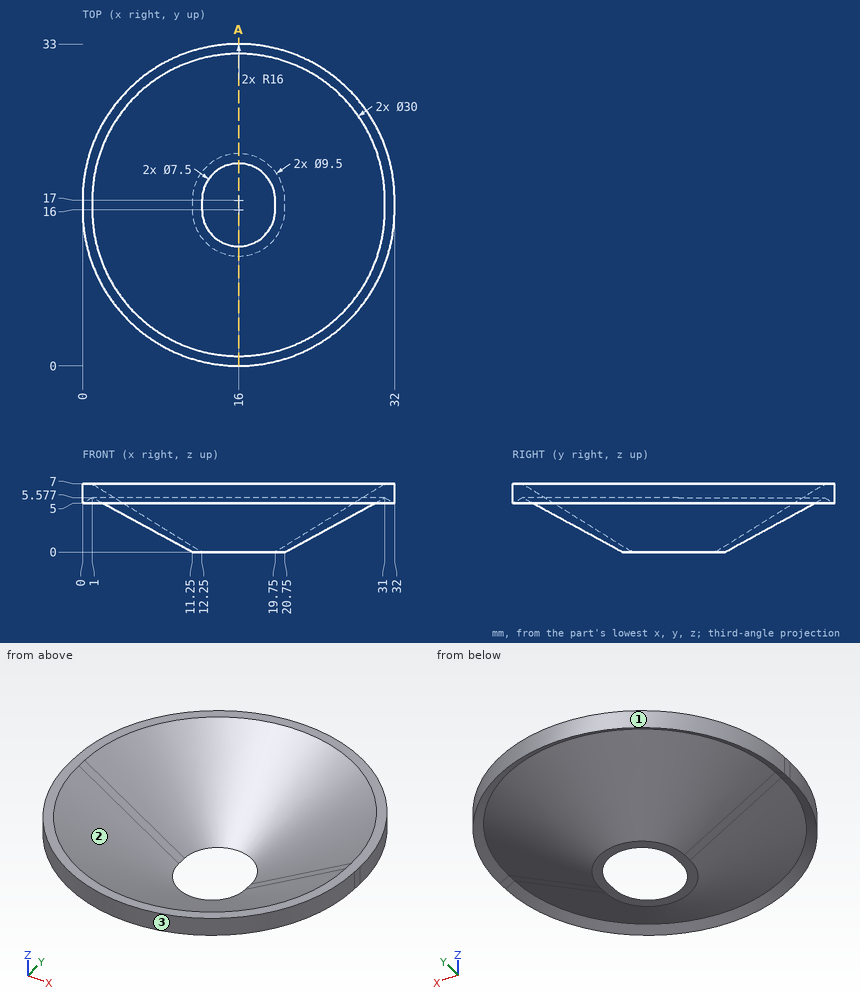
Design review of the part shown in the three views and the two pictorial views. Dimensions are in mm from the part's minimum x, y and z. Round coordinates to 2 decimals unless told otherwise and drop trailing zeros. Loops run counter-clockwise (first coordinate to the right, second up) from the corner with the lowest first, then second, coordinate; pieces in that order, holes last. Notation, with made-up numbers: (71, 52) -> (82, 52) arc R17 ccw to (82, 73) -> close; hole circle Ø1 at (33.25, 38.5). An arc over 180 degrees is marked (long way). Answer as CSV lines item,"result".
1) For P1, Ø6, axis at x = 15.5, y = 12.5, coming from the +Z side; P2, Ø1, axis at x = 12, z = 2.5, coming from the +Y side (1 decimal); P3, Ø1.5, axis at x = 21, y = 21, coming from the -Z side, all flat-tipped, find the tip position at first contact; note any pin that passes through.
Geometry results:
P1,"stops at z = 1.73"
P2,"stops at y = 26.5"
P3,"stops at z = 0.49"
2) Draft analysis for pull direction Y (two halves, no side actions). For the marked faces 1, 2 and 3, state which applies: pulls with the +Y half, pulls with the -Y half, needs draft (parallel to the pull), parting line crosses it, or undercut.
Geometry results:
face 1,"pulls with the +Y half"
face 2,"undercut"
face 3,"pulls with the -Y half"
3) To check wall thickness, follow line 1 along Y through (x, z) = (10, 4.75) (1 decimal); line 2 along X through (y, z) = (8.5, 6.75) (1 decimal); line 3 along Y through (x, z) = (17, 1.75) (1 decimal). State the ranges of each line that lie inside material, in increasing order. Write a range as from..to.
Geometry results:
line 1,"y = 3.9..6.3, 26.7..29.1"
line 2,"x = 1.9..3.5, 28.5..30.1"
line 3,"y = 8.1..9.5, 23.5..24.9"
4) Add section A-A on x = 16. Write out the cut boundary in (y, z).
Geometry results:
outline,"(0, 5) -> (1, 5.58) -> (11.25, 0) -> (12.25, 0) -> (1, 7) -> (0, 7) -> close; (20.75, 0) -> (21.75, 0) -> (32, 5.58) -> (33, 5) -> (33, 7) -> (32, 7) -> close"
